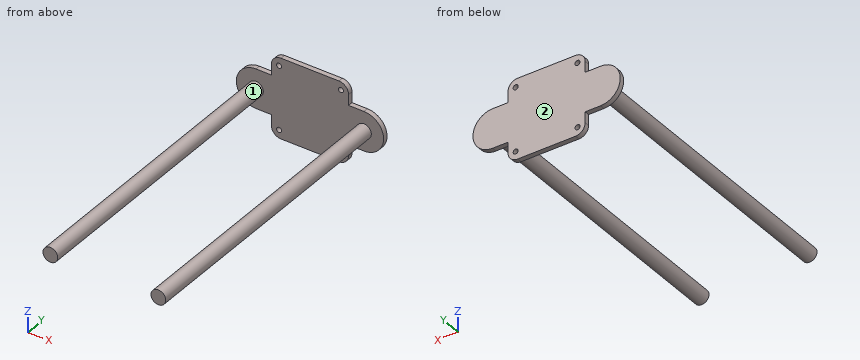
from build123d import *

# Parameters (mm, degrees)
SKETCH1_R           = 3.81
SKETCH1_W           = 39.938858144
SKETCH1_H           = 20.32
SKETCH1_R_2         = 1.3
BOSS_EXTRUDE1_DEPTH = 2.54
SKETCH1_3_R         = 3.81
BOSS_EXTRUDE2_DEPTH = 152.4


with BuildPart() as part:
    # Sketch1 → Boss-Extrude1 (new body)
    # profile 1 of 7: a face of its own
    with BuildSketch(Plane(origin=(0, 0, 0), x_dir=(1, 0, 0), z_dir=(0, 1, 0))):
        with BuildLine():
            Line((-19.969429072, -10.16), (-19.969429072, 10.16))
            Line((-19.969429072, 10.16), (-27.94, 10.16))
            ThreePointArc((-27.94, 10.16), (-38.1, 0), (-27.94, -10.16))
            Line((-27.94, -10.16), (-19.969429072, -10.16))
        make_face()
        with Locations((-27.94, 0)):
            Circle(SKETCH1_R, mode=Mode.SUBTRACT)
    # profile 2 of 7: a face of its own
    with BuildSketch(Plane(origin=(0, 0, 0), x_dir=(1, 0, 0), z_dir=(0, 1, 0))):
        Rectangle(SKETCH1_W, SKETCH1_H)
    # profile 3 of 7: a face of its own
    with BuildSketch(Plane(origin=(0, 0, 0), x_dir=(1, 0, 0), z_dir=(0, 1, 0))):
        with BuildLine():
            Line((19.969429072, -10.16), (-19.969429072, -10.16))
            Line((-19.969429072, -10.16), (-19.969429072, -15.75))
            ThreePointArc((-19.969429072, -15.75), (-18.504962978, -19.285533906), (-14.969429072, -20.75))
            Line((-14.969429072, -20.75), (14.969429072, -20.75))
            ThreePointArc((14.969429072, -20.75), (18.504962978, -19.285533906), (19.969429072, -15.75))
            Line((19.969429072, -15.75), (19.969429072, -10.16))
        make_face()
        with Locations(Location((-16, -16.5, 0), (0, 0, 270))):
            Circle(SKETCH1_R_2, mode=Mode.SUBTRACT)
        with Locations(Location((16, -16.5, 0), (0, 0, 270))):
            Circle(SKETCH1_R_2, mode=Mode.SUBTRACT)
    # profile 4 of 7: a face of its own
    with BuildSketch(Plane(origin=(0, 0, 0), x_dir=(1, 0, 0), z_dir=(0, 1, 0))):
        with BuildLine():
            Line((14.969429072, 20.75), (-14.969429072, 20.75))
            ThreePointArc((-14.969429072, 20.75), (-18.504962978, 19.285533906), (-19.969429072, 15.75))
            Line((-19.969429072, 15.75), (-19.969429072, 10.16))
            Line((-19.969429072, 10.16), (19.969429072, 10.16))
            Line((19.969429072, 10.16), (19.969429072, 15.75))
            ThreePointArc((19.969429072, 15.75), (18.504962978, 19.285533906), (14.969429072, 20.75))
        make_face()
        with Locations(Location((-16, 16.5, 0), (0, 0, 270))):
            Circle(SKETCH1_R_2, mode=Mode.SUBTRACT)
        with Locations(Location((16, 16.5, 0), (0, 0, 270))):
            Circle(SKETCH1_R_2, mode=Mode.SUBTRACT)
    # profile 5 of 7: a face of its own
    with BuildSketch(Plane(origin=(0, 0, 0), x_dir=(1, 0, 0), z_dir=(0, 1, 0))):
        with BuildLine():
            Line((27.94, 10.16), (19.969429072, 10.16))
            Line((19.969429072, 10.16), (19.969429072, -10.16))
            Line((19.969429072, -10.16), (27.94, -10.16))
            ThreePointArc((27.94, -10.16), (38.1, 0), (27.94, 10.16))
        make_face()
        with Locations((27.94, 0)):
            Circle(SKETCH1_R, mode=Mode.SUBTRACT)
    # profile 6 of 7: a face of its own
    with BuildSketch(Plane(origin=(0, 0, 0), x_dir=(1, 0, 0), z_dir=(0, 1, 0))):
        with Locations((-27.94, 0)):
            Circle(SKETCH1_R)
    # profile 7 of 7: a face of its own
    with BuildSketch(Plane(origin=(0, 0, 0), x_dir=(1, 0, 0), z_dir=(0, 1, 0))):
        with Locations((27.94, 0)):
            Circle(SKETCH1_R)
    extrude(amount=BOSS_EXTRUDE1_DEPTH)

    # Sketch1_3 → Boss-Extrude2 (add)
    with BuildSketch(Plane(origin=(0, 0, 0), x_dir=(1, 0, 0), z_dir=(0, 1, 0))):
        with Locations(Location((-27.94, 0, 0), (0, 0, 270))):
            Circle(SKETCH1_3_R)
        with Locations(Location((27.94, 0, 0), (0, 0, 270))):
            Circle(SKETCH1_3_R)
    extrude(amount=-BOSS_EXTRUDE2_DEPTH)


solid = part.part
Could you check a few things on this model? Use its own coordinates, in mm. Face numbers are marked on the shaded views. Coordinates: 2 decimals unless noted, no trailing zeros. Order: outer loops, then holes, each group sorted by start corner. A loop starts at its lowest first (then second) coordinate and runs counter-clockwise, first axis right, second up.
Q1. Suppose I cut it at D-D on z = 12.5. Please give me the cut outline in (x, y).
Q2. Will these pins go through, and if not, where does the flat tip stop? pin 1 (12 mm diameter, centred on x = 27, y = -28.5, fed in from +Z); pin 2 (3.5 mm diameter, centred on x = -16, z = 16.5, fed in from -Y); pin 3 (3 mm diameter, centred on y = 1.5, z = -12.5, fed in from -X).
Q3. Thinking about a two-plate mould opening in X: for the marked faces 1 and 2, which applies, released by +X, released by -X, zero draft, split by the parting line, or undercut?
Q4. Suppose I cut it at A-A on z = 0. Please give me the cut outline in (x, y).
Q5. Suppose I cut it at B-B on y = -132.5. Please give me the cut outline in (x, z), and give its area (3 significant figures).
Q6. Please list where these lines run through material, in increasing order: L1, parallel to Y at x = 12, z = 14; L2, parallel to X at y = 1, z = -16; L3, parallel to X at y = 0.9, z = -16.5.
Q7. Suppose I cut it at C-C on x = 1. Please give me the cut outline in (y, z), and give its area (3 significant figures).
Answer:
1. outline: (-19.97, 0) - (19.97, 0) - (19.97, 2.54) - (-19.97, 2.54) - close
2. pin 1: stops at z = 3.81
2. pin 2: stops at y = 0
2. pin 3: stops at x = -19.97
3. face 1: undercut
3. face 2: zero draft
4. outline: (-38.1, 0) - (-31.75, 0) - (-31.75, -152.4) - (-24.13, -152.4) - (-24.13, 0) - (24.13, 0) - (24.13, -152.4) - (31.75, -152.4) - (31.75, 0) - (38.1, 0) - (38.1, 2.54) - (-38.1, 2.54) - close
5. outline: circle Ø7.62 at (-27.94, 0); circle Ø7.62 at (27.94, 0)
5. area: 91.2 mm2
6. L1: y = 0 to 2.54
6. L2: x = -19.96 to -17.2, -14.8 to 14.8, 17.2 to 19.96
6. L3: x = -19.91 to -17.3, -14.7 to 14.7, 17.3 to 19.91
7. outline: (0, -20.75) - (2.54, -20.75) - (2.54, 20.75) - (0, 20.75) - close
7. area: 105 mm2
